Read the model definition and answer for the solid it produces. Units are mm, in the model's axes. A direction names the side the tool comes from. Coordinates: 2 decimals unless noted, no trailing zeros. Write each loop counter-clockwise with the first axis right and the second up, starting at its lowest first coordinate (ties: lowest second). Pieces come first, ordered by that corner, then holes. Notation, with made-up numbers: (79, 5) -> (135, 5) arc R16 cw to (135, 27) -> close; hole circle Ø5 at (-40, 35.5). An arc over 180 degrees is marked (long way). Answer as a JSON object with one key per item and string values. Group by question number.
(1) Flat-ended cylindrical pins translate along their axes: P1, Ø1.8, axis at x = 14, z = -22.5, coming from the +Y side (3 decimals); P2, Ø16, axis at x = 0, z = 0, coming from the +Y side; P3, Ø1.8, axis at x = 15, z = 14.5, coming from the +Y side (3 decimals); P4, Ø4, axis at x = -15, z = -26, coming from the +Y side. Find the tip coordinate at first contact, or state that the pin passes through.
(2) Straight lines are drawn through the part: L1, parallel to Z at x = -4, y = 12 (3 decimals); L2, parallel to X at y = 2.1, z = 0 (3 decimals); L3, parallel to X at y = 27, z = 2.5 (3 decimals). For each, find the intervals that lie inside material, in ascending order.
(3) Find section D-D (x = -15). Give the vertices of the cut face in (y, z) (1 decimal), then the cut area to 3 significant figures.
(4) For a pull along X with two mould halves and no side action, classify faces 1 (the face through (-1, 34, -31)), 2 (the face through (-19.685, 20, 0)), 3 (the face through (18, 40.1, -32)) as +X half, -X half, draft (parallel to the pull), parting line (faces both ways), or undercut.
(5) Find section A-A (z = 0). Give the vertices of the cut face in (x, y) (1 decimal).
(6) Which of the six approach directions +Z, -Z, +X, -X, +Y, -Y give full straight-line access (tool end or side, diameter ignored) to faces 4 (the face through (-9.76, 2.37, 2.17)), 5 (the face through (0, 30.9, -32)), 6 (the face through (17.091, 39.086, 32.474))?
(7) Find section B-B (y = 24). Give the vertices of the cut face in (x, z) (1 decimal).
(8) Find section C-C (x = 0). Give the vertices of the cut face in (y, z) (1 decimal), then the cut area to 3 significant figures.
from build123d import *

# Parameters (mm, degrees)
SKETCH1_W                     = 33.02
SKETCH1_H                     = 60.96
BASE_DEPTH                    = 3.175
SKETCH2_W                     = 3.51
SKETCH2_H                     = 60.96
BATTERY_SIDES_DEPTH           = 17.78
SKETCH3_W                     = 39.37
SKETCH3_H                     = 67.31
SKETCH3_W_2                   = 33.02
SKETCH3_H_2                   = 60.96
OUTER_CASING_DEPTH            = 38.1
BATTERY_PUSH_HOLE_REACH       = 56.514
SKETCH4_R                     = 10
FILLET1_R                     = 1.5875
SKETCH5_R                     = 1
ALIGNMENT_PEGS_DEPTH          = 2
ATTACHMENT_NARROW_POINT_REACH = 82.785
SKETCH6_W                     = 2
SKETCH6_H                     = 7.2
CUT_EXTRUDE4_DEPTH            = 2.157
SKETCH9_W                     = 3.51
SKETCH9_H                     = 13.97
BOSS_EXTRUDE5_DEPTH           = 6.35


with BuildPart() as part:
    # Sketch1 → Base (new body)
    with BuildSketch(Plane(origin=(0, 0, 0), x_dir=(1, 0, 0), z_dir=(0, 1, 0))):
        Rectangle(SKETCH1_W, SKETCH1_H)
        Polygon((-16.51, 30.48), (16.51, 30.48), (16.51, -30.48), align=None)
    extrude(amount=BASE_DEPTH)

    # Sketch2 → Battery-Sides (add)
    with BuildSketch(Plane(origin=(0, 3.175, 0), x_dir=(1, 0, 0), z_dir=(0, 1, 0))):
        with Locations((-14.755, 0)):
            Rectangle(SKETCH2_W, SKETCH2_H)
        with Locations((14.755, 0)):
            Rectangle(SKETCH2_W, SKETCH2_H)
    extrude(amount=BATTERY_SIDES_DEPTH)

    # Sketch3 → Outer-Casing (add)
    with BuildSketch(Plane.XZ):
        Rectangle(SKETCH3_W, SKETCH3_H)
        Rectangle(SKETCH3_W_2, SKETCH3_H_2, mode=Mode.SUBTRACT)
    extrude(amount=-OUTER_CASING_DEPTH)

    # Sketch4 → Battery-push-hole (cut, up to next)
    with BuildSketch(Plane.XZ, mode=Mode.PRIVATE) as battery_push_hole_sk1:
        with Locations(Location((0, 0, 0), (0, 0, 270))):
            Circle(SKETCH4_R)
    battery_push_hole_tool1 = extrude(battery_push_hole_sk1.sketch, amount=-BATTERY_PUSH_HOLE_REACH, mode=Mode.PRIVATE) & part.part
    add(battery_push_hole_tool1.solids().sort_by_distance((0, 0, 0))[0], mode=Mode.SUBTRACT)

    # Fillet1
    fillet1_edges = [part.edges().sort_by_distance(p)[0] for p in [
        (19.685, 19.05, 33.655),
        (19.685, 19.05, -33.655),
        (-19.685, 19.05, -33.655),
        (-19.685, 19.05, 33.655),
        (19.685, 0, 0),
        (0, 0, 33.655),
        (-19.685, 0, 0),
        (0, 0, -33.655),
        (0, 0, 10),
    ]]
    fillet(fillet1_edges, radius=FILLET1_R)

    # Sketch5 → Alignment Pegs (add)
    with BuildSketch(Plane(origin=(0, 38.1, 0), x_dir=(1, 0, 0), z_dir=(0, 1, 0))):
        with Locations(Location((-17.767235857, 31.737235857, 0), (0, 0, 90))):
            Circle(SKETCH5_R)
        with Locations(Location((-17.767235857, -31.737235857, 0), (0, 0, 90))):
            Circle(SKETCH5_R)
        with Locations(Location((17.767235857, 31.737235857, 0), (0, 0, 90))):
            Circle(SKETCH5_R)
        with Locations(Location((17.767235857, -31.737235857, 0), (0, 0, 90))):
            Circle(SKETCH5_R)
    extrude(amount=ALIGNMENT_PEGS_DEPTH)

    # Sketch6 → Attachment Narrow Point (cut, up to next)
    with BuildSketch(Plane(origin=(0, 0, -33.655), x_dir=(-1, 0, 0), z_dir=(0, 0, -1)), mode=Mode.PRIVATE) as attachment_narrow_point_sk1:
        with Locations((0, 34.5)):
            Rectangle(SKETCH6_W, SKETCH6_H)
    attachment_narrow_point_tool1 = extrude(attachment_narrow_point_sk1.sketch, amount=-ATTACHMENT_NARROW_POINT_REACH, mode=Mode.PRIVATE) & part.part
    add(attachment_narrow_point_tool1.solids().sort_by_distance((0, 34.5, -33.655))[0], mode=Mode.SUBTRACT)

    # Sketch8 → Cut-Extrude4 (cut)
    with BuildSketch(Plane.XY.offset(-33.655)):
        with BuildLine():
            ThreePointArc((1, 31.041676707), (2.877498914, 32.336669235), (3.6, 34.5))
            Line((3.6, 34.5), (3.6, 38.1))
            Line((3.6, 38.1), (1, 38.1))
            Line((1, 38.1), (1, 37.958323293))
            Line((1, 37.958323293), (1, 31.041676707))
        make_face()
        with BuildLine():
            ThreePointArc((-3.6, 34.5), (-2.877498914, 32.336669235), (-1, 31.041676707))
            Line((-1, 31.041676707), (-1, 37.958323293))
            Line((-1, 37.958323293), (-1, 38.1))
            Line((-1, 38.1), (-3.6, 38.1))
            Line((-3.6, 38.1), (-3.6, 34.5))
        make_face()
    extrude(amount=CUT_EXTRUDE4_DEPTH, mode=Mode.SUBTRACT)

    # Sketch9 → Boss-Extrude5 (add)
    with BuildSketch(Plane(origin=(0, 20.955, 0), x_dir=(1, 0, 0), z_dir=(0, 1, 0))):
        with Locations((-14.755, 23.495)):
            Rectangle(SKETCH9_W, SKETCH9_H)
        with Locations((14.755, 23.495)):
            Rectangle(SKETCH9_W, SKETCH9_H)
    extrude(amount=BOSS_EXTRUDE5_DEPTH)


solid = part.part
Results below:
{
 "1": {"P1": "stops at y = 27.305", "P2": "passes through", "P3": "stops at y = 20.955", "P4": "stops at y = 38.1"},
 "2": {"L1": "z = -33.655 to -30.48, 30.48 to 33.655", "L2": "x = -19.685 to -10, 10 to 19.685", "L3": "x = -19.685 to -16.51, 16.51 to 19.685"},
 "3": {"outline": "(0, -32.1) arc R1.6 ccw to (1.6, -33.7) -> (38.1, -33.7) -> (38.1, -30.5) -> (27.3, -30.5) -> (27.3, -16.5) -> (21, -16.5) -> (21, 30.5) -> (38.1, 30.5) -> (38.1, 33.7) -> (1.6, 33.7) arc R1.6 ccw to (0, 32.1) -> close", "area": "1,610 mm2"},
 "4": {"face 1": "undercut", "face 2": "-X half", "face 3": "draft"},
 "5": {"outline": "(-19.7, 1.6) arc R1.6 ccw to (-18.1, 0) -> (-11.6, 0) arc R1.6 ccw to (-10, 1.6) -> (-10, 3.2) -> (-13, 3.2) -> (-13, 21) -> (-16.5, 21) -> (-16.5, 38.1) -> (-19.7, 38.1) -> close; (10, 1.6) arc R1.6 ccw to (11.6, 0) -> (18.1, 0) arc R1.6 ccw to (19.7, 1.6) -> (19.7, 38.1) -> (16.5, 38.1) -> (16.5, 21) -> (13, 21) -> (13, 3.2) -> (10, 3.2) -> close"},
 "6": {"face 4": "+Y, -Y", "face 5": "-Z, +Y", "face 6": "+Y"},
 "7": {"outline": "(-19.7, -32.1) arc R1.6 ccw to (-18.1, -33.7) -> (18.1, -33.7) arc R1.6 ccw to (19.7, -32.1) -> (19.7, 32.1) arc R1.6 ccw to (18.1, 33.7) -> (-18.1, 33.7) arc R1.6 ccw to (-19.7, 32.1) -> close; hole (-16.5, -16.5) -> (-13, -16.5) -> (-13, -30.5) -> (13, -30.5) -> (13, -16.5) -> (16.5, -16.5) -> (16.5, 30.5) -> (-16.5, 30.5) -> close"},
 "8": {"outline": "(0, -32.1) arc R1.6 ccw to (1.6, -33.7) -> (30.9, -33.7) -> (30.9, -30.5) -> (3.2, -30.5) -> (3.2, -10) -> (1.6, -10) arc R1.6 ccw to (0, -11.6) -> close; (0, 11.6) arc R1.6 ccw to (1.6, 10) -> (3.2, 10) -> (3.2, 30.5) -> (38.1, 30.5) -> (38.1, 33.7) -> (1.6, 33.7) arc R1.6 ccw to (0, 32.1) -> close", "area": "347 mm2"}
}
